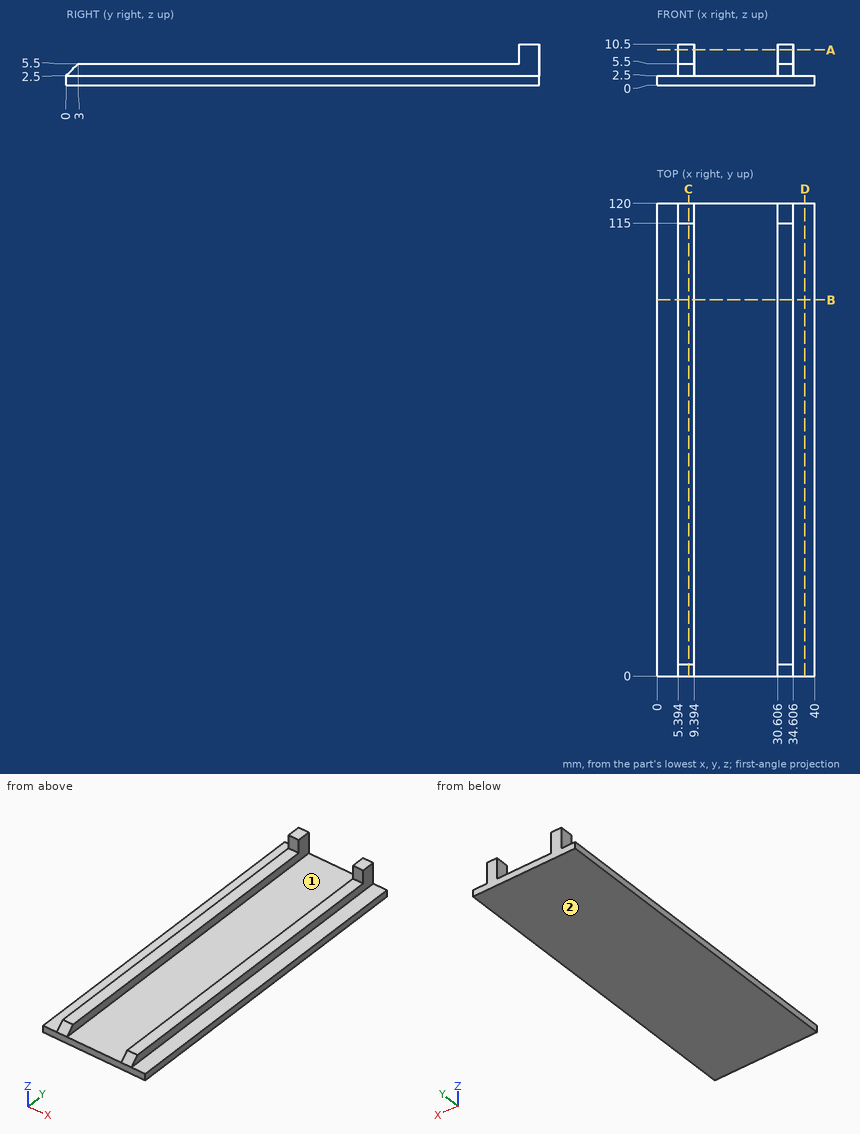
Print and shaded views of the part. All mm, measured from the part's lowest x, y and z. A direction names the side the tool comes from. Give positions to 0.01 mm unless a question says otherwise; leave off trailing zeros. Order: outer loops, then holes, each group sorted by start corner. A loop starts at its lowest first (then second) coordinate and runs counter-clockwise, first axis right, second up. Notation, with made-up numbers: (-39.75, 84) - (-31.75, 84) arc R20 cw to (-31.75, 116) - close; hole circle Ø8 at (15, 60). An arc over 180 degrees is marked (long way). One line per item, written item: value.
Item 1: Slice it at B-B (y = 95.5). List the corners of the cut face in (x, z), then the cut area to 3 significant figures.
Response values:
outline: (0, 0) - (40, 0) - (40, 2.5) - (34.61, 2.5) - (34.61, 5.5) - (30.61, 5.5) - (30.61, 2.5) - (9.39, 2.5) - (9.39, 5.5) - (5.39, 5.5) - (5.39, 2.5) - (0, 2.5) - close
area: 124 mm2
Item 2: Slice it at A-A (z = 9). List the corners of the cut face in (x, y).
Response values:
outline: (5.39, 115) - (9.39, 115) - (9.39, 120) - (5.39, 120) - close; (30.61, 115) - (34.61, 115) - (34.61, 120) - (30.61, 120) - close
Item 3: Tool access for the marked faces 1 and 2: list every direction of +Z, -Z, +X, -X, +Y, -Y with a clear straight run to the whole face (end or side of a thin tool).
Response values:
face 1: +Z, +Y, -Y
face 2: -Z, +X, -X, +Y, -Y
Item 4: Wall check: line 1 (X direction, y = 52, z = 5.25); line 2 (Z direction, x = 8, y = 63); line 3 (Z direction, x = 37.5, y = 39). Give the ranges that are in metal, low to high.
Response values:
line 1: 5.39 to 9.39, 30.61 to 34.61
line 2: 0 to 5.5
line 3: 0 to 2.5
Item 5: Pin check, flat tips, straight feed: pin 1 Ø1.2 at (x, y) = (33, 45.5) entering from +Z; pin 2 Ø8 at (x, y) = (33.5, 18.5) entering from -Z; pin 3 Ø4 at (y, z) = (64, 8) entering from -X; pin 4 Ø1.2 at (x, z) = (8, 7.5) entering from -Y. Stop position of each tip, or through.
Response values:
pin 1: z = 5.5
pin 2: z = 0
pin 3: through
pin 4: y = 115
Item 6: Slice it at C-C (x = 8). List the corners of the cut face in (y, z).
Response values:
outline: (0, 0) - (120, 0) - (120, 10.5) - (115, 10.5) - (115, 5.5) - (3, 5.5) - (0, 2.5) - close
Item 7: Slice it at D-D (x = 37.5). List the corners of the cut face in (y, z).
Response values:
outline: (0, 0) - (120, 0) - (120, 2.5) - (0, 2.5) - close
